Check sheet for the drawn part. Datum: minimum x, y, z corner. Units: mm. Coordinates: 2 decimals unless noted, no trailing zeros. Loops run counter-clockwise (first coordinate to the right, second up) from the corner with the lowest first, then second, coordinate; pieces in that order, holes last.
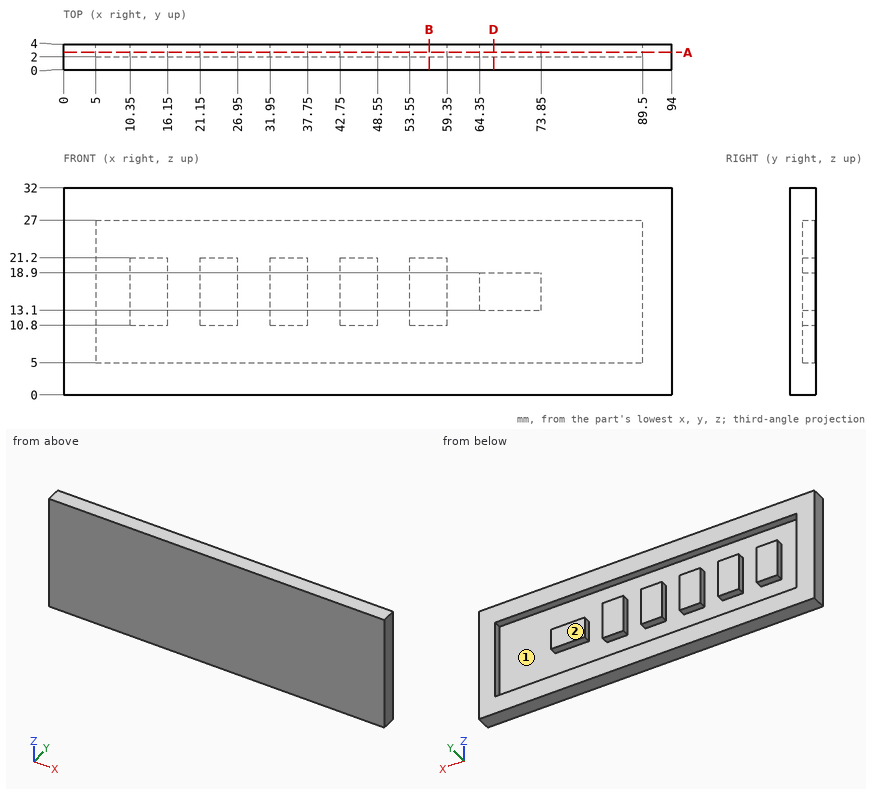
(1) Sectioned sample at D-D on x = 66.5. Record the cut outline in (y, z).
Findings:
outline: (0, 0) - (4, 0) - (4, 5) - (2, 5) - (2, 13.1) - (4, 13.1) - (4, 18.9) - (2, 18.9) - (2, 27) - (4, 27) - (4, 32) - (0, 32) - close
(2) Sectioned sample at A-A on y = 2.7. State how many separate pieces and enclosed holes the cut face has, and give its area (3 significant figures).
Findings:
separate pieces: 7
enclosed holes: 1
area: 1,510 mm2
(3) Draft check along Z on the marked faces 1 and 2. Enter one of: +Z half, -Z half, draft (parallel to the pull), parting line (faces both ways), or undercut.
Findings:
face 1: undercut
face 2: draft
(4) Scan lines: L1, parallel to Z at x = 25, y = 3.15; L2, parallel to X at y = 2.4, z = 24.5; L3, parallel to Z at x = 87, y = 2.8. Record each from-to range of solid material in increasing order.
Findings:
L1: z = 0 to 5, 10.8 to 21.2, 27 to 32
L2: x = 0 to 5, 89.5 to 94
L3: z = 0 to 5, 27 to 32
(5) Sectioned sample at B-B on x = 56.5. Record the cut outline in (y, z), and give its area (3 significant figures).
Findings:
outline: (0, 0) - (4, 0) - (4, 5) - (2, 5) - (2, 10.8) - (4, 10.8) - (4, 21.2) - (2, 21.2) - (2, 27) - (4, 27) - (4, 32) - (0, 32) - close
area: 105 mm2
